```python
from build123d import *

# Parameters (mm, degrees)
F1_W         = 70
F1_H         = 150
F2_DEPTH     = 25
F0_R         = 25
F3_DEPTH     = 150
F4_R         = 5
F5_R         = 5
F6_R         = 5
F7_T4_ANGLE  = 180
F7_T10_ANGLE = 90
F7_T16_ANGLE = 90
F8_R         = 12.5
F9_DEPTH     = 120
F10_SIZE     = 5


# Not quite as in the source:
# - a fillet or chamfer that OpenCascade refuses, or shapes differently, is made with other operations: its cross-section is extruded or revolved along the edge and cut away or added


with BuildPart() as f2:
    # F1 (on Right) → F2 (new body, symmetric)
    with BuildSketch(Plane.YZ):
        with Locations((-10, -75)):
            Rectangle(F1_W, F1_H)
    extrude(amount=F2_DEPTH, both=True)

    # F0 (on Top) → F3 (join)
    with BuildSketch(Plane.XY):
        Circle(F0_R)
    extrude(amount=F3_DEPTH)

    # F4
    f4_edges = [f2.edges().sort_by_distance(p)[0] for p in [
        (-25, 0, 150),
    ]]
    fillet(f4_edges, radius=F4_R)

    # F5
    f5_edges = [f2.edges().sort_by_distance(p)[0] for p in [
        (-25, -10, -150),
    ]]
    fillet(f5_edges, radius=F5_R)

    # F6
    f6_edges = [f2.edges().sort_by_distance(p)[0] for p in [
        (25, -10, -150),
    ]]
    fillet(f6_edges, radius=F6_R)

    # F7: chamfer of 5 on 3 edges, made by hand


with BuildPart() as f7_tool2:
    # F7_s3 → F7_t4 (revolve)
    with BuildSketch(Plane.XZ):
        Polygon((-30, 0), (-25, 5), (-25, 0), align=None)
    revolve(axis=Axis((0, 0, 0), (0, 0, 1)), revolution_arc=F7_T4_ANGLE)

    split(bisect_by=Plane.YZ.offset(25), keep=Keep.BOTTOM)

    split(bisect_by=Plane.YZ.offset(-25), keep=Keep.TOP)


with BuildPart() as f2_1:
    add(f2.part)

    # F7_t1: union F7_tool2
    add(f7_tool2.part)


with BuildPart() as f7_tool8:
    # F7_s9 → F7_t10 (revolve)
    with BuildSketch(Plane.XZ):
        Polygon((30, 0), (25, 5), (25, 0), align=None)
    revolve(axis=Axis((0, 0, 0), (0, 0, 1)), revolution_arc=F7_T10_ANGLE)

    split(bisect_by=Plane.YZ.offset(25), keep=Keep.BOTTOM)

    split(bisect_by=Plane.XZ.offset(-25), keep=Keep.TOP)


with BuildPart() as f2_2:
    add(f2_1.part)

    # F7_t7: union F7_tool8
    add(f7_tool8.part)


with BuildPart() as f7_tool14:
    # F7_s15 → F7_t16 (revolve)
    with BuildSketch(Plane.YZ):
        Polygon((30, 0), (25, 5), (25, 0), align=None)
    revolve(axis=Axis((0, 0, 0), (0, 0, 1)), revolution_arc=F7_T16_ANGLE)

    split(bisect_by=Plane.YZ.offset(-25), keep=Keep.TOP)

    split(bisect_by=Plane.XZ.offset(-25), keep=Keep.TOP)


with BuildPart() as f2_3:
    add(f2_2.part)

    # F7_t13: union F7_tool14
    add(f7_tool14.part)

    # F8 (on Front) → F9 (join)
    with BuildSketch(Plane.XZ):
        with Locations((0, -117.5)):
            Circle(F8_R)
    extrude(amount=F9_DEPTH)

    # F10
    f10_edges = [f2_3.edges().sort_by_distance(p)[0] for p in [
        (-12.5, -120, -117.5),
        (-12.5, -45, -117.5),
    ]]
    chamfer(f10_edges, length=F10_SIZE)


solid = f2_3.part
```
Source: CAD feature listing. Evaluate the final solid. Frame: model axes, mm. A direction names the side the tool comes from. Coordinates: 2 decimals unless noted, no trailing zeros. Loops run counter-clockwise (first coordinate to the right, second up) from the corner with the lowest first, then second, coordinate; pieces in that order, holes last. Notation, with made-up numbers: M 80,29.25 L 135,29.25 A34 cw 135,59.25 Z; hole C 11,-29.75 d9. An arc over 180 degrees is marked long. Use CSV: the item, a comma, the result in double quotes.
(1) Cut plane B-B on y = -33.5. Return loops of the section in (x, z), and give its area (3 significant figures).
Answers follow:
outline,"M -25,-145 A5 ccw -20,-150 L 20,-150 A5 ccw 25,-145 L 25,0 L -25,0 Z"
area,"7,490 mm²"
(2) Cut plane A-A on z = -117.5. Return loops of the section in (x, y), and give its area (4 significant figures).
Answers follow:
outline,"M -25,-45 L -17.5,-45 L -12.5,-50 L -12.5,-115 L -7.5,-120 L 7.5,-120 L 12.5,-115 L 12.5,-50 L 17.5,-45 L 25,-45 L 25,25 L -25,25 Z"
area,"5,375 mm²"
(3) Cut plane D-D on z = 109. Return loops of the section in (x, y), and give its area (3 significant figures).
Answers follow:
outline,"C 0,0 d50"
area,"1,960 mm²"
(4) Reachability of faces 1 (the face through (23.846, 7.509, 74.02)), 2 (the face through (23, 23, 0)), 3 (the face through (-1.627, -82.045, -105.106)) from +Z, -Z, +X, -X, +Y, -Y: full face, straight path, thin tool, end or side. Return the list, or none.
Answers follow:
face 1,"+Z"
face 2,"+Z, +X, +Y"
face 3,"-Y"
(5) Contact query for flat-ended pins moving along their axis: pin 1 (22.5 mm diameter, centred on x = -5.5, y = -32, fed in from +Z); pin 2 (10 mm diameter, centred on x = 8.5, z = 68, fed in from -Y); pin 3 (6.5 mm diameter, centred on x = 22.5, y = 19.5, fed in from +Z); pin 4 (5 mm diameter, centred on y = -35.5, z = 1, fed in from -X). Output: stop coordinate, or through.
Answers follow:
pin 1,"z = 149.85"
pin 2,"y = -24.75"
pin 3,"z = 3.48"
pin 4,"x = -25"
(6) Cut plane C-C on z = -50. Return loops of the section in (x, y), and give its area (3 significant figures).
Answers follow:
outline,"M -25,-45 L 25,-45 L 25,25 L -25,25 Z"
area,"3,500 mm²"
(7) Line query: line 1 (Z direction, x = 11, y = -42); line 2 (Y direction, x = 11, z = -73); line 3 (X direction, y = -73, z = -106.5). Output: solid intervals per line, ascending. Write a range as [from, to].
Answers follow:
line 1,"[-150, 0]"
line 2,"[-45, 25]"
line 3,"[-5.94, 5.94]"
